```python
from build123d import *

# Parameters (mm, degrees)
SKETCH1_W           = 44.2
SKETCH1_H           = 20
BOSS_EXTRUDE1_DEPTH = 2
SKETCH2_W           = 2
SKETCH2_H           = 20
BOSS_EXTRUDE2_DEPTH = 25
SKETCH3_R           = 3
SKETCH3_R_2         = 1.5
CUT_EXTRUDE1_DEPTH  = 25
SKETCH5_R           = 1
CUT_EXTRUDE2_DEPTH  = 56.521527357


with BuildPart() as part:
    # Sketch1 → Boss-Extrude1 (new body)
    with BuildSketch(Plane(origin=(0, 0, 0), x_dir=(1, 0, 0), z_dir=(0, 1, 0))):
        with Locations((22.1, 10)):
            Rectangle(SKETCH1_W, SKETCH1_H)
    extrude(amount=BOSS_EXTRUDE1_DEPTH)

    # Sketch2 → Boss-Extrude2 (add)
    with BuildSketch(Plane(origin=(0, 2, 0), x_dir=(1, 0, 0), z_dir=(0, 1, 0))):
        with Locations((1, 10)):
            Rectangle(SKETCH2_W, SKETCH2_H)
        with Locations((43.2, 10)):
            Rectangle(SKETCH2_W, SKETCH2_H)
    extrude(amount=BOSS_EXTRUDE2_DEPTH)

    # Sketch3 → Cut-Extrude1 (cut)
    with BuildSketch(Plane(origin=(0, 2, 0), x_dir=(1, 0, 0), z_dir=(0, 1, 0))):
        with Locations(Location((22.1, 10, 0), (0, 0, 270))):
            Circle(SKETCH3_R)
        with Locations(Location((17.1505, 14.9495, 0), (0, 0, 270))):
            Circle(SKETCH3_R_2)
        with Locations(Location((17.1505, 5.0505, 0), (0, 0, 270))):
            Circle(SKETCH3_R_2)
        with Locations(Location((27.0495, 5.0595, 0), (0, 0, 270))):
            Circle(SKETCH3_R_2)
        with Locations(Location((27.0495, 14.9495, 0), (0, 0, 270))):
            Circle(SKETCH3_R_2)
    extrude(amount=-CUT_EXTRUDE1_DEPTH, mode=Mode.SUBTRACT)

    # Sketch5 → Cut-Extrude2 (cut, through all)
    with BuildSketch(Plane.ZY):
        with Locations((-2.5, 24.5)):
            Circle(SKETCH5_R)
        with Locations((-2.779646808, 9.5)):
            Circle(SKETCH5_R)
        with Locations((-17.5, 24.5)):
            Circle(SKETCH5_R)
        with Locations((-17.779646808, 9.5)):
            Circle(SKETCH5_R)
    extrude(amount=-CUT_EXTRUDE2_DEPTH, mode=Mode.SUBTRACT)


solid = part.part
```
The model under review builds one solid part; all positions refer to its coordinate system, in mm. Give positions to 0.01 mm unless a question says otherwise; leave off trailing zeros. Loops run counter-clockwise (first coordinate to the right, second up) from the corner with the lowest first, then second, coordinate; pieces in that order, holes last. Notation, with made-up numbers: (85.5, -15.75) -> (133.5, -15.75) arc R31 ccw to (133.5, 8.25) -> close; hole circle Ø5 at (6.25, 60). An arc over 180 degrees is marked (long way). Use CSV: the item, a comma, the result in double quotes.
1. For P1, Ø10, axis at x = 32.5, y = 6.5, coming from the +Z side; P2, Ø8, axis at x = 17, z = -14.5, coming from the +Y side, all flat-tipped, find the tip position at first contact; note any pin that passes through.
Result:
P1,"stops at z = 0"
P2,"stops at y = 2"
2. Consider section D-D, the plane y = 24.5. Write out the cut boundary in (x, z), then the cut area to 3 significant figures.
Result:
outline,"(0, -20) -> (2, -20) -> (2, -18.5) -> (0, -18.5) -> close; (0, -16.5) -> (2, -16.5) -> (2, -3.5) -> (0, -3.5) -> close; (0, -1.5) -> (2, -1.5) -> (2, 0) -> (0, 0) -> close; (42.2, -20) -> (44.2, -20) -> (44.2, -18.5) -> (42.2, -18.5) -> close; (42.2, -16.5) -> (44.2, -16.5) -> (44.2, -3.5) -> (42.2, -3.5) -> close; (42.2, -1.5) -> (44.2, -1.5) -> (44.2, 0) -> (42.2, 0) -> close"
area,"64.0 mm²"
3. Consider section C-C, the plane z = -10. Write out the cut boundary in (x, y), then the cut area to 3 significant figures.
Result:
outline,"(0, 0) -> (19.1, 0) -> (19.1, 2) -> (2, 2) -> (2, 27) -> (0, 27) -> close; (25.1, 0) -> (44.2, 0) -> (44.2, 27) -> (42.2, 27) -> (42.2, 2) -> (25.1, 2) -> close"
area,"176 mm²"
4. To check wall thickness, follow probe 1 along X at (y, z) = (9, -9.75); probe 2 along Y at (x, z) = (42.6, -2.5); probe 3 along Y at (x, z) = (10, -13). State the ranges of each line that lie inside material, in increasing order. Write a range as from..to.
Result:
probe 1,"x = 0..2, 42.2..44.2"
probe 2,"y = 0..8.54, 10.46..23.5, 25.5..27"
probe 3,"y = 0..2"
5. Consider section A-A, the plane y = 6.75. Write out the cut boundary in (x, z), then the cut area to 3 significant figures.
Result:
outline,"(0, -20) -> (2, -20) -> (2, 0) -> (0, 0) -> close; (42.2, -20) -> (44.2, -20) -> (44.2, 0) -> (42.2, 0) -> close"
area,"80.0 mm²"
6. Consider section B-B, the plane x = 22.1. Write out the cut boundary in (y, z), then the cut area to 3 significant figures.
Result:
outline,"(0, -20) -> (2, -20) -> (2, -13) -> (0, -13) -> close; (0, -7) -> (2, -7) -> (2, 0) -> (0, 0) -> close"
area,"28.0 mm²"
7. The part is to be moulded in two halves that separate along X. For faces 1 (the face through (2, 14, -10)), 2 (the face through (20, 1, 0)), 3 (the face through (0, 13, -10)), say which applies: +X half, -X half, draft (parallel to the pull), parting line (faces both ways), or undercut.
Result:
face 1,"undercut"
face 2,"draft"
face 3,"-X half"
